from build123d import *

# Parameters (mm, degrees)
SKETCH1_R           = 2.3
BOSS_EXTRUDE1_DEPTH = 10.16
FILLET1_R           = 6.35
FILLET3_R           = 1


with BuildPart() as part:
    # Sketch1 → Boss-Extrude1 (new body)
    with BuildSketch(Plane.XY):
        Polygon((0, 235.981834591), (-30, 287.943358818), (-43.398894252, 287.943358818), (-43.398894252, 211.743358818), (-16.582271537, 211.743358818), (40.991016151, 244.983311963), (34.641016151, 255.981834591), align=None)
        with Locations((-37.048894252, 218.093358818)):
            Circle(SKETCH1_R, mode=Mode.SUBTRACT)
        with Locations((-37.048894252, 281.593358818)):
            Circle(SKETCH1_R, mode=Mode.SUBTRACT)
        with Locations((32.316754837, 247.307573277)):
            Circle(SKETCH1_R, mode=Mode.SUBTRACT)
        with Locations((-11.677335675, 221.907573277)):
            Circle(SKETCH1_R, mode=Mode.SUBTRACT)
    extrude(amount=BOSS_EXTRUDE1_DEPTH)

    # Fillet1
    fillet1_edges = [part.edges().sort_by_distance(p)[0] for p in [
        (-30, 287.943358818, 5.08),
        (-16.582271537, 211.743358818, 5.08),
        (-43.398894252, 211.743358818, 5.08),
        (-43.398894252, 287.943358818, 5.08),
        (34.641016151, 255.981834591, 5.08),
        (40.991016151, 244.983311963, 5.08),
        (0, 235.981834591, 5.08),
    ]]
    fillet(fillet1_edges, radius=FILLET1_R - 0.0001)  # a hair under: the kernel refuses the full size

    # Fillet3
    fillet3_edges = [part.edges().sort_by_distance(p)[0] for p in [
        (-15.670945881, 263.124709061, 0),
        (-15.670945881, 263.124709061, 10.16),
        (17.320508076, 245.981834591, 0),
        (17.320508076, 245.981834591, 10.16),
        (10.191534663, 227.201223035, 0),
        (-27.666358183, 211.743358818, 0),
        (-43.398894252, 249.843358818, 0),
        (-35.357555363, 287.943358818, 0),
        (-41.539051602, 286.083516168, 0),
        (-41.539051602, 213.603201469, 0),
        (-16.640247059, 211.959726414, 0),
        (-30.491166474, 287.09263353, 0),
        (38.450423844, 245.66406162, 0),
        (33.960266494, 253.441242284, 0),
        (-35.357555363, 287.943358818, 10.16),
        (-43.398894252, 249.843358818, 10.16),
        (-27.666358183, 211.743358818, 10.16),
        (10.191534663, 227.201223035, 10.16),
        (-41.539051602, 286.083516168, 10.16),
        (-41.539051602, 213.603201469, 10.16),
        (-16.640247059, 211.959726414, 10.16),
        (-30.491166474, 287.09263353, 10.16),
        (38.450423844, 245.66406162, 10.16),
        (33.960266494, 253.441242284, 10.16),
        (0.680749657, 238.522426898, 0),
        (0.680749657, 238.522426898, 10.16),
    ]]
    fillet(fillet3_edges, radius=FILLET3_R)


solid = part.part
Input: part model. Units: mm. Frame: model coordinates. A direction names the side the tool comes from. Give positions to 0.01 mm unless a question says otherwise; leave off trailing zeros. Use one line per item in the form item = value.
1. First-contact query: P1, Ø3, axis at x = 6.5, z = 4.5, coming from the +Y side; P2, Ø1, axis at y = 249, z = 8.5, coming from the +X side; P3, Ø3, axis at x = -37.05, y = 281.59, coming from the -Z side (1 decimal); P4, Ø1.5, axis at x = 14, z = 9, coming from the -Y side. Flat tips, straight axial feed; report the tip coordinate or a pass-through.
Outcome:
P1 = 240.6
P2 = 38.55
P3 = through
P4 = 228.97
2. Cut plane A-A on z = 6. State how many separate pieces and enclosed holes the cut face has, and give its area (3 significant figures).
Outcome:
separate_pieces = 1
enclosed_holes = 4
area = 2,910 mm²
3. Ray query, L1, parallel to Y at x = 31.5, z = 2; L2, parallel to X at y = 224.5, z = 8.25; L3, parallel to X at y = 242, z = 1.25. Return the intervals inside material, ascending.
Outcome:
L1 = 239.5 to 245.16, 249.46 to 253.6
L2 = -43.4 to 5.51
L3 = -43.4 to -3.47, 10.42 to 35.8
4. Mould query, pull axis X, two halves, no side actions, for faces 5 (the face through (-41.588, 213.653, 5.137)), 6 (the face through (38.468, 245.732, 5.137)), 7 (the face through (-12.176, 219.662, 5.009)), 8 (the face through (17.49, 246.08, 5.02)). Classes: released by +X, released by -X, zero draft, split by the parting line, or undercut.
Outcome:
face_5 = released by -X
face_6 = released by +X
face_7 = undercut
face_8 = undercut
5. Reachability of faces 1 (the face through (17.3, 245.64, 0.3)), 2 (the face through (17.3, 245.64, 9.86)), 3 (the face through (-21, 242, 10.16)), 4 (the face through (-15.496, 262.822, 5.023)) from +Z, -Z, +X, -X, +Y, -Y: full face, straight path, thin tool, end or side. Return the list, or none.
Outcome:
face_1 = -Z, +Y
face_2 = +Z, +Y
face_3 = +Z, +X, -X, +Y, -Y
face_4 = +Z, -Z, +Y
